Input: part model. Units: mm. Frame: model coordinates. A direction names the side the tool comes from. Give positions to 0.01 mm unless a question says otherwise; leave off trailing zeros. Loops run counter-clockwise (first coordinate to the right, second up) from the corner with the lowest first, then second, coordinate; pieces in that order, holes last. Notation, with made-up numbers: M 13.25,-1.5 L 38.25,-1.5 A27 ccw 38.25,27.5 Z; hole C -35.5,-4 d11. An arc over 180 degrees is marked long. Answer as a JSON object with one key per item and string values. Group by question number.
1) Ray query, L1, parallel to X at y = -4.75, z = 46.5; L2, parallel to Z at x = -36.5, y = -5.75; L3, parallel to X at y = -4, z = -28. Return the intervals inside material, ascending.
2) Access query for faces 1 (the flat face through (-112.3, -12.52, 11.98)), 2 (the flat face through (-66.88, -13.81, -72.31)), 3 (the flat face through (121, -13, -46.885)). Directions: +Z, -Z, +X, -X, +Y, -Y. A direction counts if a zero-diameter tool reaches every point of the face in a straight line with its end or side. Return the directions, or none.
3) Section query B-B on z = -29. Return loops of the section in (x, y).
4) First-contact query: P1, Ø11.5, axis at y = -9, z = -14.5, coming from the -X side; P2, Ø8, axis at y = -22.5, z = -52.5, coming from the -X side; P3, Ø5, axis at x = 111.5, y = -5, coming from the -Z side. Flat tips, straight axial feed; report the tip coordinate or a pass-through.
5) Draft query along Z for faces 4 (the flat face through (-67.446, -12.522, -74.805)), 5 (the flat face through (25, -14, 78.499)), 6 (the flat face through (-112.303, -12.522, 63.135)). Return one class per face: +Z half, -Z half, draft (parallel to the pull), parting line (faces both ways), or undercut.
6) Section query A-A on x = 36. Return loops of the section in (y, z), plus the area to 3 significant figures.
from build123d import *

# Parameters (mm, degrees)
F1_DEPTH = 25.4
F2_T     = -2.54


with BuildPart() as f1:
    # F0 (on Front) → F1 (new body)
    with BuildSketch(Plane.XZ):
        Polygon((-49.9549284577, -57.7479749918), (-49.9549284577, 57.7479749918), (-84.4545662403, 57.7479749918), (-84.4545662403, 14.6633386612), (-84.4545662403, -14.6633386612), (-84.4545662403, -57.7479749918), align=None)
        Polygon((-84.4545662403, 57.7479749918), (-84.4545662403, 68.7423571944), (-140.9429758787, 57.3688596487), align=None)
        Polygon((-84.4545662403, -14.6633386612), (-84.4545662403, 14.6633386612), (-140.9429758787, 9.2210201547), (-140.9429758787, -9.2210201547), align=None)
        Polygon((-140.9429758787, -57.3688596487), (-84.4545662403, -68.7423571944), (-84.4545662403, -57.7479749918), align=None)
        Polygon((-84.4545662403, -68.7423571944), (-49.9549284577, -81.0392451267), (-49.9549284577, -57.7479749918), (-84.4545662403, -57.7479749918), align=None)
        Polygon((0, -81.0392451267), (0, 81.0392451267), (-49.9549284577, 81.0392451267), (-49.9549284577, 57.7479749918), (-49.9549284577, -57.7479749918), (-49.9549284577, -81.0392451267), align=None)
        Polygon((99.88479051, 81.0392451267), (0, 81.0392451267), (0, -81.0392451267), (100.1753211021, -81.0392451267), (100.1140988569, -46.8851514161), (99.9460127552, 46.8851514161), align=None)
        Polygon((141.5084600449, 46.8851514161), (99.9460127552, 46.8851514161), (100.1140988569, -46.8851514161), (141.5084600449, -46.8851514161), (141.5084600449, 0), align=None)
        Polygon((-49.9549284577, 57.7479749918), (-49.9549284577, 81.0392451267), (-84.4545662403, 68.7423571944), (-84.4545662403, 57.7479749918), align=None)
    extrude(amount=F1_DEPTH)

    # F2
    f2_openings = [f1.faces().sort_by_distance(p)[0] for p in [
        (14.722317, -25.4, -0.014513),
    ]]
    offset(amount=F2_T, openings=f2_openings, kind=Kind.INTERSECTION)


solid = f1.part
Output:
{
 "1": {"L1": "x = -84.45 to -81.91, 97.41 to 141.51", "L2": "z = -81.04 to -78.5, 78.5 to 81.04", "L3": "x = -84.45 to -81.91, 138.97 to 141.51"},
 "2": {"face 1": "-X, +Y, -Y", "face 2": "-Y", "face 3": "-Z, +X, +Y, -Y"},
 "3": {"outline": "M -84.45,-25.4 L -81.91,-25.4 L -81.91,-2.54 L 138.97,-2.54 L 138.97,-25.4 L 141.51,-25.4 L 141.51,0 L -84.45,0 Z"},
 "4": {"P1": "stops at x = -140.94", "P2": "stops at x = -84.45", "P3": "stops at z = -46.89"},
 "5": {"face 4": "-Z half", "face 5": "undercut", "face 6": "+Z half"},
 "6": {"outline": "M -25.4,-81.04 L 0,-81.04 L 0,81.04 L -25.4,81.04 L -25.4,78.5 L -2.54,78.5 L -2.54,-78.5 L -25.4,-78.5 Z", "area": "528 mm^2"}
}
